from build123d import *

# Parameters (mm, degrees)
F0_R     = 50
F1_DEPTH = 50
F2_R     = 17.5
F3_DEPTH = 45
F4_R     = 5
F5_R     = 17.5
F6_DEPTH = 50.001
F7_T     = -1.5


with BuildPart() as f1:
    # F0 (on Front) → F1 (new body)
    with BuildSketch(Plane.XZ):
        with BuildLine():
            ThreePointArc((14, -58.3438085833), (47.1168759576, -37.148351242), (60, 0))
            ThreePointArc((60, 0), (47.1168759576, 37.148351242), (14, 58.3438085833))
            ThreePointArc((14, 58.3438085833), (-60, 0), (14, -58.3438085833))
        make_face()
        Circle(F0_R, mode=Mode.SUBTRACT)
        with BuildLine():
            ThreePointArc((14, 58.3438085833), (47.1168759576, 37.148351242), (60, 0))
            ThreePointArc((60, 0), (47.1168759576, -37.148351242), (14, -58.3438085833))
            Line((14, -58.3438085833), (155.8333333333, -24.309920243))
            ThreePointArc((155.8333333333, -24.309920243), (125, 0), (155.8333333333, 24.309920243))
            Line((155.8333333333, 24.309920243), (14, 58.3438085833))
        make_face()
        with BuildLine():
            ThreePointArc((175, 0), (169.632031649, 15.4784796842), (155.8333333333, 24.309920243))
            ThreePointArc((155.8333333333, 24.309920243), (125, 0), (155.8333333333, -24.309920243))
            ThreePointArc((155.8333333333, -24.309920243), (169.632031649, -15.4784796842), (175, 0))
        make_face()
    extrude(amount=F1_DEPTH)

    # F5 (on face) → F6 (cut, through all)
    with BuildSketch(Plane.XZ.offset(50)):
        with Locations((150, 0)):
            Circle(F5_R)
    extrude(amount=-F6_DEPTH, mode=Mode.SUBTRACT)

    # F7
    f7_openings = [f1.faces().sort_by_distance(p)[0] for p in [
        (65.769085, -50, 0),
    ]]
    offset(amount=F7_T, openings=f7_openings)



with BuildPart() as f3:
    # F2 (on face) → F3 (new body)
    with BuildSketch(Plane(origin=(14, 0, 58.3438085833), x_dir=(0.9723968097, 0, -0.2333333333), z_dir=(0.2333333333, 0, 0.9723968097))):
        with Locations((72.9297607291, -25)):
            Circle(F2_R)
    extrude(amount=F3_DEPTH)

    # F4
    f4_edges = [f3.edges().sort_by_distance(p)[0] for p in [
        (78.399722, -25, 89.168054),
        (67.899722, -25, 45.410198),
    ]]
    fillet(f4_edges, radius=F4_R)


with BuildPart() as f1_1:
    add(f1.part)

    add(f3.part)  # F8 merges F3
    # F8: F3 across plane
    add(f3.part.mirror(Plane.XY))


solid = f1_1.part
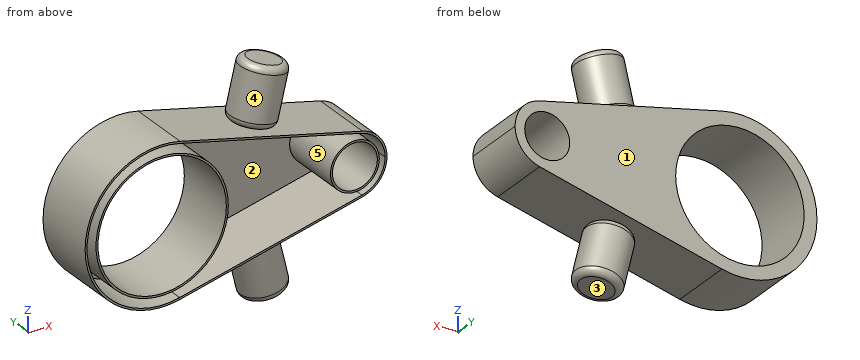
Verification items for the finished model (mm, model axes). Face numbers are marked on the shaded views. A direction names the side the tool comes from. Round coordinates to 2 decimals unless told otherwise and drop trailing zeros. Loops run counter-clockwise (first coordinate to the right, second up) from the corner with the lowest first, then second, coordinate; pieces in that order, holes last. Notation, with made-up numbers: (-18.75, -2) - (38.25, -2) arc R29 ccw to (38.25, 35) - close; hole circle Ø10 at (-27, 14). An arc over 180 degrees is marked (long way). Use one line per item in the form item = value.
1. Section check B-B on z = 30.5. Record the cut outline in (x, y).
A:
outline = (-51.67, -50) - (-49.92, -50) - (-49.92, -1.5) - (-41.5, -1.5) - (-41.5, -50) - (-39.62, -50) - (-39.62, 0) - (-51.67, 0) - close; (39.62, -50) - (41.5, -50) - (41.5, -1.5) - (123.61, -1.5) - (123.61, -50) - (130.04, -50) - (130.04, 0) - (39.62, 0) - close
2. Scan lines: probe 1 along Z at (x, y) = (0, -18); probe 2 along Z at (x, y) = (-45, -35.5); probe 3 along X at (y, z) = (-27, 6.5). Record each from-to range of solid material in increasing order.
A:
probe_1 = -60 to -58.5, -51.5 to -50, 50 to 51.5, 58.5 to 60
probe_2 = -39.69 to -37.38, -25.04 to -21.79, 21.79 to 25.04, 37.38 to 39.69
probe_3 = -59.65 to -58.14, -51.09 to -49.58, 49.58 to 51.09, 132.15 to 133.75, 166.25 to 167.85, 172.58 to 174.14
3. Draft check along Z on the marked faces 1, 2 and 3. Enter one of: pulls with the +Z half, pulls with the -Z half, needs draft (parallel to the pull), parting line crosses it, or undercut.
A:
face_1 = needs draft
face_2 = undercut
face_3 = pulls with the -Z half
4. Gauge pin test, flat ends, axial feed: pin 1 Ø8 at (x, z) = (113, 5.5) entering from +Y; pin 2 Ø5 at (x, y) = (42, -9.5) entering from +Z; pin 3 Ø10 at (y, z) = (-6, -70.5) entering from -X; pin 4 Ø8 at (y, z) = (-14, -66.5) entering from +X. Record the tip position at first contact, or that the pin passes through.
A:
pin_1 = 0
pin_2 = 52.22
pin_3 = 81.02
pin_4 = 107.68
5. Section check C-C on y = -15.5. Give the number of separate pieces and of enclosed holes in the cut face, and give its area (3 significant figures).
A:
separate_pieces = 3
enclosed_holes = 3
area = 4,100 mm²
6. Section check A-A on x = 0. Record the cut outline in (y, z), and give its area (3 significant figures).
A:
outline = (-50, -60) - (0, -60) - (0, -50) - (-50, -50) - (-50, -51.5) - (-1.5, -51.5) - (-1.5, -58.5) - (-50, -58.5) - close; (-50, 50) - (0, 50) - (0, 60) - (-50, 60) - (-50, 58.5) - (-1.5, 58.5) - (-1.5, 51.5) - (-50, 51.5) - close
area = 321 mm²
7. Access from +Z, -Z, +X, -X, +Y, -Y to the whole of each face (thin tool, end or side, straight path). Record for the marked faces 4 and 5.
A:
face_4 = none
face_5 = -Y
